Geometry check sheet. Reference: the model listing, model coordinates, mm. Face numbers are marked on the shaded views. A direction names the side the tool comes from. Coordinates: 2 decimals unless noted, no trailing zeros. Write each loop counter-clockwise with the first axis right and the second up, starting at its lowest first coordinate (ties: lowest second). Pieces come first, ordered by that corner, then holes. Notation, with made-up numbers: M -23.5,32 L -17.5,32 A27 ccw -17.5,48 Z; hole C 44,71.5 d8. An arc over 180 degrees is marked long. Write each question's results on one line, items separated by ' | '.
```python
from build123d import *

# Parameters (mm, degrees)
SKETCH1_W                 = 27
SKETCH1_H                 = 17
SKETCH1_W_2               = 23
SKETCH1_H_2               = 13
BOSS_EXTRUDE1_DEPTH       = 1.5
SKETCH1_3_W               = 27
SKETCH1_3_H               = 17
SKETCH1_3_W_2             = 23
SKETCH1_3_H_2             = 13
BOSS_EXTRUDE2_DEPTH       = 17
SKETCH2_W                 = 4.291322887
SKETCH2_H                 = 2.933386364
CUT_EXTRUDE1_DEPTH        = 14.5
SKETCH3_R                 = 1.776145291
CUT_EXTRUDE2_DEPTH        = 14.5
SKETCH4_W                 = 17
SKETCH4_H                 = 17
BOSS_EXTRUDE3_DEPTH       = 5
SKETCH5_W                 = 6.111771398
SKETCH5_H                 = 16.943398975
BOSS_EXTRUDE4_DEPTH       = 23
SKETCH6_R                 = 1.5
BOSS_EXTRUDE9_DEPTH       = 22
SKETCH10_W                = 10.152493364
SKETCH10_H                = 16.970590483
BOSS_EXTRUDE10_DEPTH      = 3
BOSS_EXTRUDE10_DEPTH_BACK = 23
SKETCH8_W                 = 5.111825198
SKETCH8_H                 = 22.20816513
CUT_EXTRUDE4_DEPTH        = 3
CUT_EXTRUDE4_DEPTH_BACK   = 3
SKETCH11_R                = 1.55
CUT_EXTRUDE5_DEPTH        = 31


with BuildPart() as part:
    # Sketch1 → Boss-Extrude1 (new body)
    with BuildSketch(Plane(origin=(0, 0, 0), x_dir=(1, 0, 0), z_dir=(0, 1, 0))):
        Rectangle(SKETCH1_W, SKETCH1_H)
        Rectangle(SKETCH1_W_2, SKETCH1_H_2, mode=Mode.SUBTRACT)
        Rectangle(SKETCH1_W_2, SKETCH1_H_2)
    extrude(amount=BOSS_EXTRUDE1_DEPTH)

    # Sketch1<3> → Boss-Extrude2 (add)
    with BuildSketch(Plane(origin=(0, 0, 0), x_dir=(1, 0, 0), z_dir=(0, 1, 0))):
        Rectangle(SKETCH1_3_W, SKETCH1_3_H)
        Rectangle(SKETCH1_3_W_2, SKETCH1_3_H_2, mode=Mode.SUBTRACT)
    extrude(amount=BOSS_EXTRUDE2_DEPTH)

    # Sketch2 → Cut-Extrude1 (cut)
    with BuildSketch(Plane(origin=(0, 17, 0), x_dir=(1, 0, 0), z_dir=(0, 1, 0))):
        with Locations((12.620499192, 0)):
            Rectangle(SKETCH2_W, SKETCH2_H)
    extrude(amount=-CUT_EXTRUDE1_DEPTH, mode=Mode.SUBTRACT)

    # Sketch3 → Cut-Extrude2 (cut)
    with BuildSketch(Plane(origin=(0, 1.5, 0), x_dir=(1, 0, 0), z_dir=(0, 1, 0))):
        with Locations(Location((-6.765421027, 0, 0), (0, 0, 270))):
            Circle(SKETCH3_R)
    cut_extrude2 = extrude(amount=-CUT_EXTRUDE2_DEPTH, mode=Mode.SUBTRACT)

    # Mirror1: Cut-Extrude2 across plane
    add(cut_extrude2.mirror(Plane(origin=(0, 0, 0), x_dir=(0, 0, 1), z_dir=(1, 0, 0))), mode=Mode.SUBTRACT)

    # Sketch4 → Boss-Extrude3 (add)
    with BuildSketch(Plane.ZY.offset(13.5)):
        with Locations((0, 8.5)):
            Rectangle(SKETCH4_W, SKETCH4_H)
    extrude(amount=BOSS_EXTRUDE3_DEPTH)

    # Sketch5 → Boss-Extrude4 (add)
    with BuildSketch(Plane.XZ):
        with Locations((-21.555885699, -0.028300512)):
            Rectangle(SKETCH5_W, SKETCH5_H)
    extrude(amount=-BOSS_EXTRUDE4_DEPTH)



with BuildPart() as body_2:
    # Sketch6 → Boss-Extrude9 (new body)
    with BuildSketch(Plane(origin=(0, 23, 0), x_dir=(1, 0, 0), z_dir=(0, 1, 0))):
        with BuildLine():
            Line((-19.397979401, -13.709269216), (-19.397979401, -8.443398975))
            Line((-19.397979401, -8.443398975), (-13.397979401, -8.5))
            Line((-13.397979401, -8.5), (-13.397979401, -13.709269216))
            ThreePointArc((-13.397979401, -13.709269216), (-16.397979401, -16.709269216), (-19.397979401, -13.709269216))
        make_face()
        with Locations(Location((-16.397979401, -13.709269216, 0), (0, 0, 180))):
            Circle(SKETCH6_R, mode=Mode.SUBTRACT)
    extrude(amount=-BOSS_EXTRUDE9_DEPTH)


with BuildPart() as part_1:
    add(part.part)

    add(body_2.part)  # Boss-Extrude10 merges body 2
    # Sketch10 → Boss-Extrude10 (add, two sides)
    with BuildSketch(Plane(origin=(0, 23, 0), x_dir=(1, 0, 0), z_dir=(0, 1, 0))) as boss_extrude10_sk:
        with Locations((-21.591786232, 0.014704758)):
            Rectangle(SKETCH10_W, SKETCH10_H)
    extrude(amount=BOSS_EXTRUDE10_DEPTH)
    extrude(boss_extrude10_sk.sketch, amount=-BOSS_EXTRUDE10_DEPTH_BACK)

    # Sketch8 → Cut-Extrude4 (cut, two sides)
    with BuildSketch(Plane(origin=(0, 26, 0), x_dir=(1, 0, 0), z_dir=(0, 1, 0))) as cut_extrude4_sk:
        with Locations((-21.223699311, -0.490089781)):
            Rectangle(SKETCH8_W, SKETCH8_H)
    extrude(amount=CUT_EXTRUDE4_DEPTH, mode=Mode.SUBTRACT)
    extrude(cut_extrude4_sk.sketch, amount=-CUT_EXTRUDE4_DEPTH_BACK, mode=Mode.SUBTRACT)

    # Sketch11 → Cut-Extrude5 (cut)
    with BuildSketch(Plane(origin=(0, 23, 0), x_dir=(1, 0, 0), z_dir=(0, 1, 0))):
        with Locations(Location((-16.397979401, -13.709269216, 0), (0, 0, 180))):
            Circle(SKETCH11_R)
    extrude(amount=-CUT_EXTRUDE5_DEPTH, mode=Mode.SUBTRACT)


solid = part_1.part
```
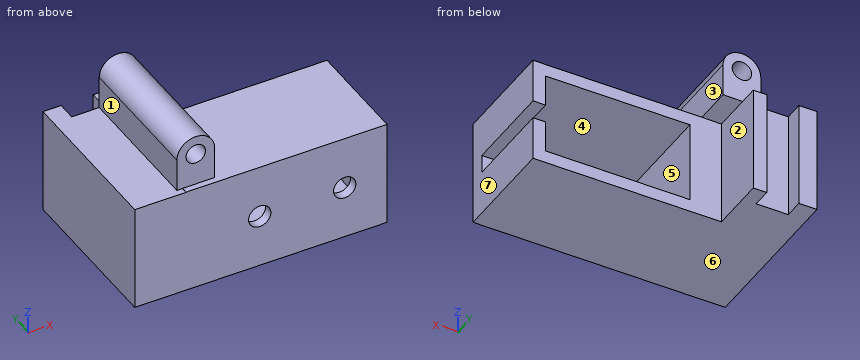
Q1. Sectioned sample at A-A on z = 0. Record the cut outline in (x, y), and give its area (3 significant figures).
Geometry check:
outline: M -26.67,0 L -8.54,0 L -8.54,1.5 L -11.5,1.5 L -11.5,17 L -16.52,17 L -16.52,26 L -18.67,26 L -18.67,23 L -23.78,23 L -23.78,26 L -26.67,26 Z; M -4.99,0 L 4.99,0 L 4.99,1.5 L -4.99,1.5 Z; M 8.54,0 L 13.5,0 L 13.5,2.5 L 11.5,2.5 L 11.5,1.5 L 8.54,1.5 Z | area: 363 mm2
Q2. Sectioned sample at C-C on x = -1. Record the cut outline in (y, z), and give its area (3 significant figures).
Geometry check:
outline: M 0,-8.5 L 17,-8.5 L 17,-6.5 L 1.5,-6.5 L 1.5,6.5 L 17,6.5 L 17,8.5 L 0,8.5 Z | area: 87.5 mm2
Q3. Sectioned sample at B-B on y = 17.5. Record the cut outline in (x, z).
Geometry check:
outline: M -26.67,-8.5 L -16.52,-8.5 L -16.52,8.47 L -13.4,8.5 L -13.4,13.71 A3 ccw -19.4,13.71 L -19.4,8.47 L -26.67,8.47 Z; hole C -16.4,13.71 d3.1
Q4. Access from +Z, -Z, +X, -X, +Y, -Y to the whole of each face (thin tool, end or side, straight path). Record for the marked faces 1, 2 and 3.
Geometry check:
face 1: +Z, -X, +Y, -Y | face 2: -Z, +X, +Y | face 3: +Z, +X, +Y, -Y
Q5. Sectioned sample at D-D on y = 14.25. Record the cut outline in (x, z).
Geometry check:
outline: M -26.67,-8.5 L 13.5,-8.5 L 13.5,-1.47 L 11.5,-1.47 L 11.5,-6.5 L -11.5,-6.5 L -11.5,6.5 L 11.5,6.5 L 11.5,1.47 L 13.5,1.47 L 13.5,8.5 L -13.4,8.5 L -13.4,13.71 A3 ccw -19.4,13.71 L -19.4,8.47 L -26.67,8.47 Z; hole C -16.4,13.71 d3.1
Q6. Depth check by flat-ended pin: P1, Ø1.5, axis at x = -15, z = 12.5, coming from the -Y side; P2, Ø10, axis at x = -3.5, y = 6, coming from the +Z side; P3, Ø4, axis at y = 14, z = 11.5, coming from the -X side. Enter the tip coordinate at first touch or a pass-through.
Geometry check:
P1: stops at y = 1 | P2: stops at z = 8.5 | P3: stops at x = -19.4
Q7. Scan lines: probe 1 along X at (y, z) = (5.75, 2.75); probe 2 along X at (y, z) = (0.95, 0); probe 3 along Z at (x, y) = (-4, 8.5). Record each from-to range of solid material in increasing order.
Geometry check:
probe 1: x = -26.67 to -11.5, 11.5 to 13.5 | probe 2: x = -26.67 to -8.54, -4.99 to 4.99, 8.54 to 13.5 | probe 3: z = -8.5 to -6.5, 6.5 to 8.5
Q8. Mould release check, pull along Z, two halves, no side actions. Record for the marked faces 4, 5, 6 and 7: pulls with the +Z half, pulls with the -Z half, needs draft (parallel to the pull), parting line crosses it, or undercut.
Geometry check:
face 4: undercut | face 5: undercut | face 6: pulls with the -Z half | face 7: needs draft
